```python
from build123d import *

# Parameters (mm, degrees)
F0_R     = 25
F0_R_2   = 1.25
F1_DEPTH = 3


with BuildPart() as f1:
    # F0 (on Top) → F1 (new body)
    with BuildSketch(Plane.XY):
        Circle(F0_R)
        with Locations((-15, -15)):
            Circle(F0_R_2, mode=Mode.SUBTRACT)
        with Locations((-10, -20)):
            Circle(F0_R_2, mode=Mode.SUBTRACT)
        with Locations((-5, -20)):
            Circle(F0_R_2, mode=Mode.SUBTRACT)
        with Locations((-10, -15)):
            Circle(F0_R_2, mode=Mode.SUBTRACT)
        with Locations((-5, -15)):
            Circle(F0_R_2, mode=Mode.SUBTRACT)
        with Locations((-20, -10)):
            Circle(F0_R_2, mode=Mode.SUBTRACT)
        with Locations((-15, -10)):
            Circle(F0_R_2, mode=Mode.SUBTRACT)
        with Locations((-20, -5)):
            Circle(F0_R_2, mode=Mode.SUBTRACT)
        with Locations((-15, -5)):
            Circle(F0_R_2, mode=Mode.SUBTRACT)
        with Locations((-10, -10)):
            Circle(F0_R_2, mode=Mode.SUBTRACT)
        with Locations((-5, -10)):
            Circle(F0_R_2, mode=Mode.SUBTRACT)
        with Locations((-10, -5)):
            Circle(F0_R_2, mode=Mode.SUBTRACT)
        with Locations((-5, -5)):
            Circle(F0_R_2, mode=Mode.SUBTRACT)
        with Locations((0, -20)):
            Circle(F0_R_2, mode=Mode.SUBTRACT)
        with Locations((5, -20)):
            Circle(F0_R_2, mode=Mode.SUBTRACT)
        with Locations((10, -20)):
            Circle(F0_R_2, mode=Mode.SUBTRACT)
        with Locations((0, -15)):
            Circle(F0_R_2, mode=Mode.SUBTRACT)
        with Locations((5, -15)):
            Circle(F0_R_2, mode=Mode.SUBTRACT)
        with Locations((10, -15)):
            Circle(F0_R_2, mode=Mode.SUBTRACT)
        with Locations((15, -15)):
            Circle(F0_R_2, mode=Mode.SUBTRACT)
        with Locations((0, -10)):
            Circle(F0_R_2, mode=Mode.SUBTRACT)
        with Locations((5, -10)):
            Circle(F0_R_2, mode=Mode.SUBTRACT)
        with Locations((10, -10)):
            Circle(F0_R_2, mode=Mode.SUBTRACT)
        with Locations((0, -5)):
            Circle(F0_R_2, mode=Mode.SUBTRACT)
        with Locations((5, -5)):
            Circle(F0_R_2, mode=Mode.SUBTRACT)
        with Locations((10, -5)):
            Circle(F0_R_2, mode=Mode.SUBTRACT)
        with Locations((15, -10)):
            Circle(F0_R_2, mode=Mode.SUBTRACT)
        with Locations((20, -10)):
            Circle(F0_R_2, mode=Mode.SUBTRACT)
        with Locations((15, -5)):
            Circle(F0_R_2, mode=Mode.SUBTRACT)
        with Locations((20, -5)):
            Circle(F0_R_2, mode=Mode.SUBTRACT)
        with Locations((-20, 0)):
            Circle(F0_R_2, mode=Mode.SUBTRACT)
        with Locations((-20, 5)):
            Circle(F0_R_2, mode=Mode.SUBTRACT)
        with Locations((-15, 0)):
            Circle(F0_R_2, mode=Mode.SUBTRACT)
        with Locations((-15, 5)):
            Circle(F0_R_2, mode=Mode.SUBTRACT)
        with Locations((-20, 10)):
            Circle(F0_R_2, mode=Mode.SUBTRACT)
        with Locations((-15, 10)):
            Circle(F0_R_2, mode=Mode.SUBTRACT)
        with Locations((-10, 0)):
            Circle(F0_R_2, mode=Mode.SUBTRACT)
        with Locations((-10, 5)):
            Circle(F0_R_2, mode=Mode.SUBTRACT)
        with Locations((-5, 0)):
            Circle(F0_R_2, mode=Mode.SUBTRACT)
        with Locations((-5, 5)):
            Circle(F0_R_2, mode=Mode.SUBTRACT)
        with Locations((-10, 10)):
            Circle(F0_R_2, mode=Mode.SUBTRACT)
        with Locations((-5, 10)):
            Circle(F0_R_2, mode=Mode.SUBTRACT)
        with Locations((-15, 15)):
            Circle(F0_R_2, mode=Mode.SUBTRACT)
        with Locations((-10, 15)):
            Circle(F0_R_2, mode=Mode.SUBTRACT)
        with Locations((-5, 15)):
            Circle(F0_R_2, mode=Mode.SUBTRACT)
        with Locations((-10, 20)):
            Circle(F0_R_2, mode=Mode.SUBTRACT)
        with Locations((-5, 20)):
            Circle(F0_R_2, mode=Mode.SUBTRACT)
        Circle(F0_R_2, mode=Mode.SUBTRACT)
        with Locations((5, 0)):
            Circle(F0_R_2, mode=Mode.SUBTRACT)
        with Locations((0, 5)):
            Circle(F0_R_2, mode=Mode.SUBTRACT)
        with Locations((5, 5)):
            Circle(F0_R_2, mode=Mode.SUBTRACT)
        with Locations((10, 0)):
            Circle(F0_R_2, mode=Mode.SUBTRACT)
        with Locations((10, 5)):
            Circle(F0_R_2, mode=Mode.SUBTRACT)
        with Locations((0, 10)):
            Circle(F0_R_2, mode=Mode.SUBTRACT)
        with Locations((5, 10)):
            Circle(F0_R_2, mode=Mode.SUBTRACT)
        with Locations((10, 10)):
            Circle(F0_R_2, mode=Mode.SUBTRACT)
        with Locations((15, 0)):
            Circle(F0_R_2, mode=Mode.SUBTRACT)
        with Locations((15, 5)):
            Circle(F0_R_2, mode=Mode.SUBTRACT)
        with Locations((20, 0)):
            Circle(F0_R_2, mode=Mode.SUBTRACT)
        with Locations((20, 5)):
            Circle(F0_R_2, mode=Mode.SUBTRACT)
        with Locations((15, 10)):
            Circle(F0_R_2, mode=Mode.SUBTRACT)
        with Locations((20, 10)):
            Circle(F0_R_2, mode=Mode.SUBTRACT)
        with Locations((0, 15)):
            Circle(F0_R_2, mode=Mode.SUBTRACT)
        with Locations((5, 15)):
            Circle(F0_R_2, mode=Mode.SUBTRACT)
        with Locations((10, 15)):
            Circle(F0_R_2, mode=Mode.SUBTRACT)
        with Locations((0, 20)):
            Circle(F0_R_2, mode=Mode.SUBTRACT)
        with Locations((5, 20)):
            Circle(F0_R_2, mode=Mode.SUBTRACT)
        with Locations((10, 20)):
            Circle(F0_R_2, mode=Mode.SUBTRACT)
        with Locations((15, 15)):
            Circle(F0_R_2, mode=Mode.SUBTRACT)
    extrude(amount=F1_DEPTH)


solid = f1.part
```
For this review, take the finished solid that the model builds, in its own axes (mm). Round coordinates to 2 decimals unless told otherwise and drop trailing zeros. Write each loop counter-clockwise with the first axis right and the second up, starting at its lowest first coordinate (ties: lowest second). Pieces come first, ordered by that corner, then holes. Notation, with made-up numbers: (59.25, -6) - (118.25, -6) arc R21 cw to (118.25, 3) - close; hole circle Ø7 at (2.25, 34). An arc over 180 degrees is marked (long way). Put each result on its own line as item: value.
Q1. Mouldability with a two-part tool opening along X and no side actions: class faces 1 (the face through (23.846, 7.509, 1.479)), 2 (the face through (-18.845, -0.479, 1.479)), 3 (the face through (-5.27, 18.78, 1.48)) as released by +X, released by -X, zero draft, split by the parting line, or undercut.
Solved:
face 1: split by the parting line
face 2: undercut
face 3: undercut
Q2. Wall thickness on probe 1 along Y at (x, z) = (-20, 1.05); probe 2 along X at (y, z) = (-22.5, 0.25); probe 3 along Y at (x, z) = (-3, 0.2): over which ranges is each line inside the solid? List them lowest first.
Solved:
probe 1: y = -15 to -11.25, -8.75 to -6.25, -3.75 to -1.25, 1.25 to 3.75, 6.25 to 8.75, 11.25 to 15
probe 2: x = -10.9 to 10.9
probe 3: y = -24.82 to 24.82
Q3. We need section A-A (x = 15). Count the separate pieces of the cut face and the enclosed holes in it, and give its area (3 significant figures).
Solved:
separate pieces: 8
enclosed holes: 0
area: 67.5 mm2
Q4. Insertion check: pin 1 Ø1 at (y, z) = (-12.5, 1.5) entering from +X; pin 2 Ø4 at (x, y) = (-4, -19.5) entering from +Z; pin 3 Ø1 at (y, z) = (-7, 1.5) entering from -X; pin 4 Ø1.5 at (y, z) = (-3.5, 1.5) entering from -X. Each pin has a flat end and moves straight along its axis. Give the tip position at first contact, or say it passes through.
Solved:
pin 1: stops at x = 21.93
pin 2: stops at z = 3
pin 3: stops at x = -24.14
pin 4: stops at x = -24.85
Q5. We need section C-C (x = 20). Give the boundary of the cut face in (y, z).
Solved:
outline: (-15, 0) - (-11.25, 0) - (-11.25, 3) - (-15, 3) - close; (-8.75, 0) - (-6.25, 0) - (-6.25, 3) - (-8.75, 3) - close; (-3.75, 0) - (-1.25, 0) - (-1.25, 3) - (-3.75, 3) - close; (1.25, 0) - (3.75, 0) - (3.75, 3) - (1.25, 3) - close; (6.25, 0) - (8.75, 0) - (8.75, 3) - (6.25, 3) - close; (11.25, 0) - (15, 0) - (15, 3) - (11.25, 3) - close
